Design review of the part built by this model. Coordinates are the model's own, in mm. A direction names the side the tool comes from. Give positions to 0.01 mm unless a question says otherwise; leave off trailing zeros. Loops run counter-clockwise (first coordinate to the right, second up) from the corner with the lowest first, then second, coordinate; pieces in that order, holes last. Notation, with made-up numbers: (-14, -32) - (31, -32) arc R33 cw to (31, 5) - close; hole circle Ø2 at (-25, 44). An arc over 180 degrees is marked (long way). Write each question's results on one line, items separated by ' | '.
from build123d import *

# Parameters (mm, degrees)
BOSS_EXTRUDE1_DEPTH = 66
SKETCH3_W           = 2
SKETCH3_H           = 8
CUT_EXTRUDE1_DEPTH  = 37
SKETCH3_3_W         = 2
SKETCH3_3_H         = 8
BOSS_EXTRUDE2_DEPTH = 29
BOSS_EXTRUDE3_REACH = 58
SKETCH4_W           = 12
SKETCH4_H           = 42
SKETCH4_W_2         = 10
SKETCH5_W           = 12
SKETCH5_H           = 6
CUT_EXTRUDE2_DEPTH  = 25


with BuildPart() as part:
    # Sketch2 → Boss-Extrude1 (new body)
    with BuildSketch(Plane.XY):
        Polygon((0, 0), (12, 0), (12, -42), (113.8, -42), (113.8, 0), (125.8, 0), (125.8, -42), (169.8, -42), (169.8, 0), (181.8, 0), (181.8, -57), (0, -57), align=None)
    extrude(amount=-BOSS_EXTRUDE1_DEPTH)

    # Sketch3 → Cut-Extrude1 (cut)
    with BuildSketch(Plane.XY):
        with Locations((11, -21)):
            Rectangle(SKETCH3_W, SKETCH3_H)
    extrude(amount=-CUT_EXTRUDE1_DEPTH, mode=Mode.SUBTRACT)

    # Sketch3_3 → Boss-Extrude2 (add)
    with BuildSketch(Plane.XY):
        with Locations((11, -21)):
            Rectangle(SKETCH3_3_W, SKETCH3_3_H)
    extrude(amount=-BOSS_EXTRUDE2_DEPTH)

    # Sketch4 → Boss-Extrude3 (add, up to next)
    with BuildSketch(Plane(origin=(125.8, 0, 0), x_dir=(0, 0, -1), z_dir=(1, 0, 0)), mode=Mode.PRIVATE) as boss_extrude3_sk1:
        with Locations((6, -21)):
            Rectangle(SKETCH4_W, SKETCH4_H)
    boss_extrude3_tool1 = extrude(boss_extrude3_sk1.sketch, amount=BOSS_EXTRUDE3_REACH, mode=Mode.PRIVATE) - part.part
    add(boss_extrude3_tool1.solids().sort_by_distance((125.8, -21, -6))[0])
    # Sketch4 → Boss-Extrude3 (add, up to next)
    with BuildSketch(Plane(origin=(125.8, 0, 0), x_dir=(0, 0, -1), z_dir=(1, 0, 0)), mode=Mode.PRIVATE) as boss_extrude3_sk2:
        with Locations((61, -21)):
            Rectangle(SKETCH4_W_2, SKETCH4_H)
    boss_extrude3_tool2 = extrude(boss_extrude3_sk2.sketch, amount=BOSS_EXTRUDE3_REACH, mode=Mode.PRIVATE) - part.part
    add(boss_extrude3_tool2.solids().sort_by_distance((125.8, -21, -61))[0])

    # Sketch5 → Cut-Extrude2 (cut)
    with BuildSketch(Plane(origin=(0, 0, 0), x_dir=(1, 0, 0), z_dir=(0, 1, 0))):
        with Locations((119.8, 34)):
            Rectangle(SKETCH5_W, SKETCH5_H)
    extrude(amount=-CUT_EXTRUDE2_DEPTH, mode=Mode.SUBTRACT)


solid = part.part
(1) Take a section at D-D on z = -18. Give the boundary of the cut face in (x, y).
Answers below:
outline: (0, -57) - (181.8, -57) - (181.8, 0) - (169.8, 0) - (169.8, -42) - (125.8, -42) - (125.8, 0) - (113.8, 0) - (113.8, -42) - (12, -42) - (12, 0) - (0, 0) - close
(2) Take a section at C-C on x = 142. Give the boundary of the cut face in (y, z), plus the area to 3 significant figures.
Answers below:
outline: (-57, -66) - (0, -66) - (0, -56) - (-42, -56) - (-42, -12) - (0, -12) - (0, 0) - (-57, 0) - close | area: 1,910 mm2
(3) Insertion check: P1, Ø3, axis at x = 119, z = -34, coming from the +Y side; P2, Ø13, axis at x = 140.5, z = -43, coming from the +Y side. Each pin has a flat end and moves straight along its axis. Give the tip position at first contact, or say it passes through.
Answers below:
P1: y = -25 | P2: y = -42
(4) Draft analysis for pull direction Z (two halves, no side actions). For faces 4 (the flat face through (110, -48, -66)), 5 (the flat face through (147, 0, -11)), 6 (the flat face through (147, -21, -12)), state which applies: pulls with the +Z half, pulls with the -Z half, needs draft (parallel to the pull), parting line crosses it, or undercut.
Answers below:
face 4: pulls with the -Z half | face 5: needs draft | face 6: undercut
(5) Wall thickness on line 1 along X through (y, z) = (-14, -54); line 2 along X through (y, z) = (-37, -5); line 3 along Z through (x, y) = (167.5, -33.5): over which ranges is each line inside the solid? List them lowest first. Write a range as from..to.
Answers below:
line 1: 0..12, 113.8..125.8, 169.8..181.8 | line 2: 0..12, 113.8..181.8 | line 3: -66..-56, -12..0
(6) Take a section at A-A on y = -14. Give the boundary of the cut face in (x, z).
Answers below:
outline: (0, -66) - (12, -66) - (12, 0) - (0, 0) - close; (113.8, -66) - (181.8, -66) - (181.8, 0) - (113.8, 0) - (113.8, -31) - (125.8, -31) - (125.8, -12) - (169.8, -12) - (169.8, -56) - (125.8, -56) - (125.8, -37) - (113.8, -37) - close
(7) Take a section at B-B on z = -62. Give the boundary of the cut face in (x, y), plus the area to 3 significant figures.
Answers below:
outline: (0, -57) - (181.8, -57) - (181.8, 0) - (113.8, 0) - (113.8, -42) - (12, -42) - (12, 0) - (0, 0) - close | area: 6,090 mm2
(8) Tool access review of faces 1 (the flat face through (125.8, -25.4, -33.7)), 2 (the flat face through (10, -21, -33)), 3 (the flat face through (113.8, -26, -33)): name each direction out of +Z, -Z, +X, -X, +Y, -Y from which nothing blocks a thin tool from reaching the whole face with its end or side.
Answers below:
face 1: +Y | face 2: none | face 3: +Z, -Z, +Y
